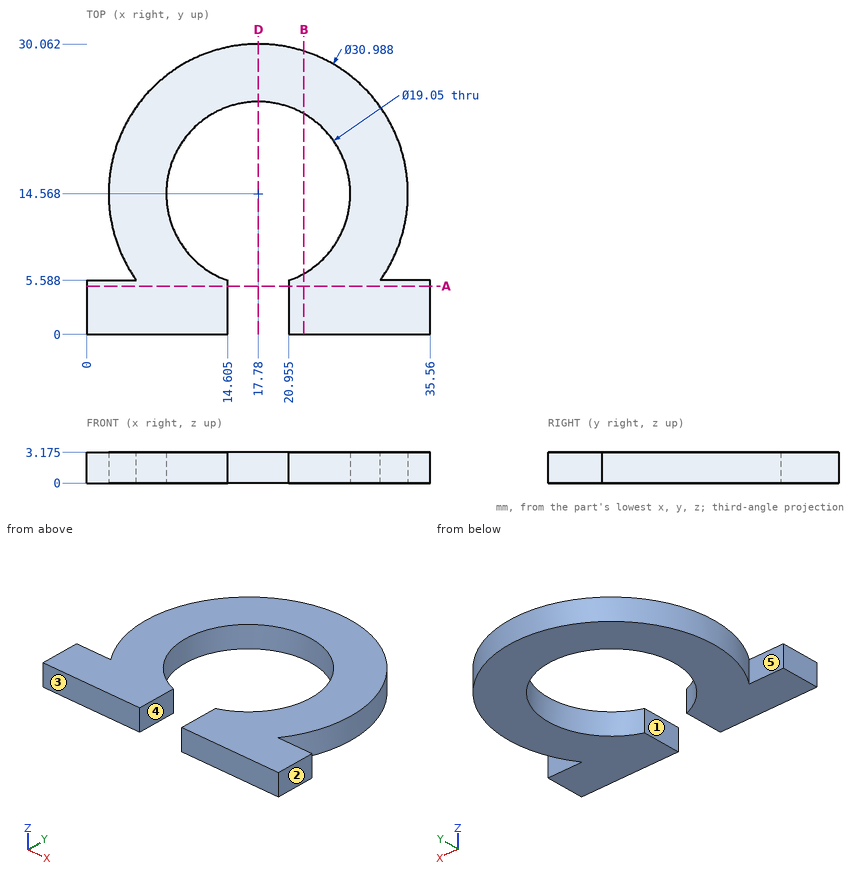
Can you work these out from the drawing? Everything is in mm from the part's minimum corner. A direction names the side the tool comes from. Give positions to 0.01 mm unless a question says otherwise; leave off trailing zeros. Order: outer loops, then holes, each group sorted by start corner. A loop starts at its lowest first (then second) coordinate and runs counter-clockwise, first axis right, second up. Notation, with made-up numbers: M 55,-4.5 L 61,-4.5 A14 ccw 61,3.5 Z; hole C 57.25,-3 d2. An arc over 180 degrees is marked long. Use a Markdown table: item, result. Add a question column.
1. On a 3-axis mill with a long thin cutter (end or side, diameter ignored), from which of +Z, -Z, +X, -X, +Y, -Y can I reach the whole of each face in a straight line? I mean the marked faces 1 and 2. Say none if no direction works.
2. Suppose I cut it at D-D (x = 17.78). List the corners of the cut face in (y, z) for me (1 decimal).
3. Suppose I cut it at B-B (x = 22.5). List the corners of the cut face in (y, z) for me (1 decimal).
4. I need wall thicknesses on probe 1 along X at (y, z) = (5, 2.85) (1 decimal); probe 2 along Y at (x, z) = (30, 3) (1 decimal); probe 3 along X at (y, z) = (16.5, 2.2). Which ranges of each line are inside material? Lowest first, please. Write a range as from..to.
5. Suppose I cut it at A-A (y = 5). List the corners of the cut face in (x, z) for me (1 decimal).
6. If we mould it in two halves opening along Y, with no side actions, what happens to the marked faces 3, 4 and 5? For each: +Y half, -Y half, draft (parallel to the pull), parting line (faces both ways), or undercut.
7. For pin 1 Ø1.6 at (x, z) = (3, 1.5) entering from +Y, with a flat end and sliding along its axis, tell me the tip position at first contact or that it passes through.
Results list:
| question | item | result |
|---|---|---|
| 1 | face 1 | +Z, -Z, -Y |
| 1 | face 2 | +Z, -Z, +X, +Y, -Y |
| 2 | outline | M 24.1,0 L 30.1,0 L 30.1,3.2 L 24.1,3.2 Z |
| 3 | outline | M 0,0 L 6.3,0 L 6.3,3.2 L 0,3.2 Z; M 22.8,0 L 29.3,0 L 29.3,3.2 L 22.8,3.2 Z |
| 4 | probe 1 | x = 0..14.6, 21..35.6 |
| 4 | probe 2 | y = 0..24.1 |
| 4 | probe 3 | x = 2.41..8.45, 27.11..33.15 |
| 5 | outline | M 0,0 L 14.6,0 L 14.6,3.2 L 0,3.2 Z; M 21,0 L 35.6,0 L 35.6,3.2 L 21,3.2 Z |
| 6 | face 3 | -Y half |
| 6 | face 4 | draft |
| 6 | face 5 | undercut |
| 7 | pin 1 | stops at y = 21.25 |
